Design review of the part built by this model. Coordinates are the model's own, in mm. Face numbers are marked on the shaded views. A direction names the side the tool comes from. Coordinates: 2 decimals unless noted, no trailing zeros. Write each loop counter-clockwise with the first axis right and the second up, starting at its lowest first coordinate (ties: lowest second). Pieces come first, ordered by that corner, then holes. Notation, with made-up numbers: (71, -16) - (110, -16) arc R15 ccw to (110, 7) - close; hole circle Ø9 at (-27, -38). An arc over 180 degrees is marked (long way). One line per item, written item: value.
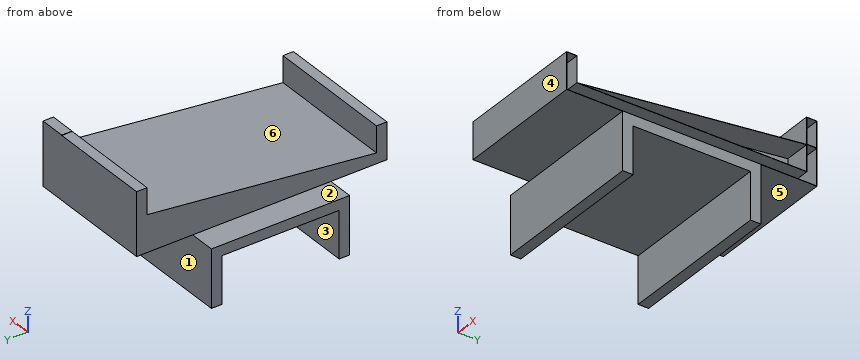
from build123d import *

# Parameters (mm, degrees)
F1_DEPTH = 15
F2_DEPTH = 10
F4_DEPTH = 5
F0_W     = 2
F0_H     = 5
F5_DEPTH = 10
F6_DEPTH = 10
F3_W     = 1.9
F3_H     = 4.95
F7_DEPTH = 5


with BuildPart() as f1:
    # F0 (on Right) → F1 (new body, symmetric)
    with BuildSketch(Plane.YZ):
        Polygon((-11.25, 4.5), (11.25, 4.5), (11.25, -4.5), (13.25, -4.5), (13.25, 6.5), (-13.25, 6.5), (-13.25, -4.5), (-11.25, -4.5), align=None)
    extrude(amount=F1_DEPTH, both=True)

    # F0 (on Right) → F2 (join, symmetric)
    with BuildSketch(Plane.YZ):
        Polygon((-13.25, 6.5), (13.25, 6.5), (24, 6.5), (24, 13.5), (22, 13.5), (22, 8.5), (-22, 8.5), (-22, 13.5), (-24, 13.5), (-24, 6.5), align=None)
    extrude(amount=F2_DEPTH, both=True)

    # F3 (on face) → F4 (join)
    with BuildSketch(Plane.YZ.offset(10)):
        Polygon((-22, 13.5), (-24, 13.5), (-24, 6.5), (-13.25, 6.5), (13.25, 6.5), (24, 6.5), (24, 13.5), (23.95, 13.5), (23.95, 6.55), (-23.95, 6.55), (-23.95, 13.45), (-22.05, 13.45), (-22.05, 8.45), (22.05, 8.45), (22.05, 13.5), (22, 13.5), (22, 13.4496782049), (22.0004976757, 13.449734759), (22, 8.5), (-21.5571682035, 8.5), (-22, 8.5), align=None)
    extrude(amount=F4_DEPTH)

    # F0 (on Right) → F5 (join, symmetric)
    with BuildSketch(Plane.YZ):
        with Locations((23, 16)):
            Rectangle(F0_W, F0_H)
    extrude(amount=F5_DEPTH, both=True)

    # F0 (on Right) → F6 (join, symmetric)
    with BuildSketch(Plane.YZ):
        Polygon((22, 8.5), (22, 13.5), (-22, 8.5), align=None)
    extrude(amount=F6_DEPTH, both=True)

    # F3 (on face) → F7 (join)
    with BuildSketch(Plane.YZ.offset(10)):
        Polygon((22, 18.5646470636), (22, 13.5), (22.05, 13.5), (23.95, 13.5), (24, 13.5), (24, 18.5646470636), align=None)
        with Locations((23, 16.0396470636)):
            Rectangle(F3_W, F3_H, mode=Mode.SUBTRACT)
        Polygon((22, 13.5), (-22, 8.5), (-21.5571682035, 8.5), (22, 13.4496782049), align=None)
    extrude(amount=F7_DEPTH)


solid = f1.part
1. Consider section A-A, the plane x = 11.75. Give the number of separate pieces and of enclosed holes in the cut face, then the cut area to 3 significant figures.
Answer block:
separate pieces: 1
enclosed holes: 3
area: 97.8 mm^2
2. Consider section C-C, the plane x = 4. Write out the cut boundary in (y, z), then the cut area to 3 significant figures.
Answer block:
outline: (-24, 6.5) - (-13.25, 6.5) - (-13.25, -4.5) - (-11.25, -4.5) - (-11.25, 4.5) - (11.25, 4.5) - (11.25, -4.5) - (13.25, -4.5) - (13.25, 6.5) - (24, 6.5) - (24, 18.5) - (22, 18.5) - (22, 13.5) - (-22, 8.5) - (-22, 13.5) - (-24, 13.5) - close
area: 325 mm^2
3. Insertion check: pin 1 Ø7 at (x, z) = (-6.5, 0) entering from -Y; pin 2 Ø0.6 at (x, y) = (8.5, -23) entering from +Z; pin 3 Ø0.6 at (y, z) = (23.5, 16) entering from +X. Each pin has a flat end and moves straight along its axis. Give the tip position at first contact, or say it passes through.
Answer block:
pin 1: stops at y = -13.25
pin 2: stops at z = 13.5
pin 3: stops at x = 10
4. Consider section D-D, the plane z = 15. Write out the cut boundary in (x, y).
Answer block:
outline: (-10, 22) - (15, 22) - (15, 22.05) - (10, 22.05) - (10, 23.95) - (15, 23.95) - (15, 24) - (-10, 24) - close
5. Wall thickness on line 1 along Y through (x, z) = (6.75, -3.25); line 2 along Y through (x, z) = (-6, 17.5); line 3 along X through (y, z) = (-8, 9): over which ranges is each line inside the solid? List them lowest first.
Answer block:
line 1: y = -13.25 to -11.25, 11.25 to 13.25
line 2: y = 22 to 24
line 3: x = -10 to 10
6. For the marked faces 1, 2 and 3, list the 3-axis set-ups (+Z, -Z, +X, -X, +Y, -Y) from which the entire face can be reached by the end or side of a thin tool; tool diameter is ignored.
Answer block:
face 1: -Z, +X, -X, +Y
face 2: +Z, -X, +Y, -Y
face 3: -Z, +X, -X
7. Mouldability with a two-part tool opening along Y and no side actions: class the marked faces 4, 5 and 6 as released by +Y, released by -Y, zero draft, split by the parting line, or undercut.
Answer block:
face 4: released by -Y
face 5: zero draft
face 6: undercut
8. Consider section B-B, the plane z = -1. Write out the cut boundary in (x, y), then the cut area to 3 significant figures.
Answer block:
outline: (-15, -13.25) - (15, -13.25) - (15, -11.25) - (-15, -11.25) - close; (-15, 11.25) - (15, 11.25) - (15, 13.25) - (-15, 13.25) - close
area: 120 mm^2
